```python
from build123d import *

# Parameters (mm, degrees)
F0_W = 10
F0_H = 6


with BuildPart() as f1:
    # F0 (on Top) → F1 (revolve)
    with BuildSketch(Plane.XY):
        Polygon((0, 0), (25, 0), (25, 12.5), (25, 15), (0, 15), align=None)
        Polygon((25, 0), (40, 0), (40, 10), (40, 12.5), (25, 12.5), align=None)
        Polygon((40, 0), (55, 0), (55, 8), (55, 10), (40, 10), align=None)
        Polygon((55, 0), (70, 0), (70, 6), (70, 8), (55, 8), align=None)
        with Locations((75, 3)):
            Rectangle(F0_W, F0_H)
    revolve(axis=Axis((32.5, 0, 0), (1, 0, 0)))


solid = f1.part
```
The model under review builds one solid part; all positions refer to its coordinate system, in mm. A direction names the side the tool comes from. Round coordinates to 2 decimals unless told otherwise and drop trailing zeros. Loops run counter-clockwise (first coordinate to the right, second up) from the corner with the lowest first, then second, coordinate; pieces in that order, holes last. Notation, with made-up numbers: (73, 32.25) - (97, 32.25) arc R31 ccw to (97, 62.25) - close; hole circle Ø6 at (4.5, 86.5). An arc over 180 degrees is marked (long way). Use a Markdown table: item, result. Add a question column.
Q1. Add section C-C (x = 18). State the section outline as (y, z) points, plus the area to 3 significant figures.
Q2. Insertion check: pin 1 Ø8 at (x, y) = (36, 11.5) entering from +Z; pin 2 Ø5 at (y, z) = (-4.5, 6.5) entering from -X; pin 3 Ø1 at (x, y) = (30.5, -11) entering from -Z; pin 4 Ø1.5 at (x, y) = (56.5, -4.5) entering from -Z. Each pin has a flat end and moves straight along its axis. Give the tip position at first contact, or say it passes through.
Q3. Machinability: for faces 1 (the face through (47.4, -2.17, -9.76)), 2 (the face through (0, 0, 0)), which of the approach directions +Z, -Z, +X, -X, +Y, -Y give a long, thin tool a straight path to every point of the face, cutting with its end or side? Answer none if there is none.
Q4. Add section A-A (z = 0). State the section outline as (x, y) points.
Q5. Add section D-D (x = 38). State the section outline as (y, z) points.
Q6. For probe 1 along X at (y, z) = (4, 13.25); probe 2 along X at (y, z) = (-9.25, 3.5); probe 3 along Y at (x, z) = (14.5, 12.5), list the stretches that pass through material, from the lowest coordinate up.
Worked answers:
| question | item | result |
|---|---|---|
| 1 | outline | circle Ø30 at (0, 0) |
| 1 | area | 707 mm² |
| 2 | pin 1 | z = 10 |
| 2 | pin 2 | x = 0 |
| 2 | pin 3 | z = -6.78 |
| 2 | pin 4 | z = -7.07 |
| 3 | face 1 | +X |
| 3 | face 2 | +Z, -Z, -X, +Y, -Y |
| 4 | outline | (0, -15) - (25, -15) - (25, -12.5) - (40, -12.5) - (40, -10) - (55, -10) - (55, -8) - (70, -8) - (70, -6) - (80, -6) - (80, 6) - (70, 6) - (70, 8) - (55, 8) - (55, 10) - (40, 10) - (40, 12.5) - (25, 12.5) - (25, 15) - (0, 15) - close |
| 5 | outline | circle Ø25 at (0, 0) |
| 6 | probe 1 | 0 to 25 |
| 6 | probe 2 | 0 to 55 |
| 6 | probe 3 | -8.29 to 8.29 |
